Read the model definition and answer for the solid it produces. Units are mm, in the model's axes. Face numbers are marked on the shaded views. Coordinates: 2 decimals unless noted, no trailing zeros. Order: outer loops, then holes, each group sorted by start corner. A loop starts at its lowest first (then second) coordinate and runs counter-clockwise, first axis right, second up.
Autodesk Inventor part; units mm, degrees
ref_plane "YZ Plane" through (0, 0, 0) normal (1, 0, 0) x (0, 1, 0)
ref_plane "XZ Plane" through (0, 0, 0) normal (0, 1, 0) x (-1, 0, 0)
ref_plane "XY Plane" through (0, 0, 0) normal (0, 0, 1) x (1, 0, 0)
sketch "Sketch1" plane through (0, 0, 0) normal (0, 0, 1) x (1, 0, 0)
  line L0 (-3, 0) -> (3, 0) construction
  line L1 (-3, -1.5) -> (3, -1.5)
  line L2 (3, 1.5) -> (-3, 1.5)
  arc A0 (-3, 1.5) -> (-3, -1.5) centre (-3, 0) ccw
  arc A1 (3, -1.5) -> (3, 1.5) centre (3, 0) ccw
  point P0 (0, 0)
  point P1 (4.5, 0)
  point P2 (-4.5, 0)
  dimension "d0" = 3
  dimension "d1" = 9
extrude "Extrusion1" add sketch "Sketch1" along normal blind 7.5
sketch "Sketch2" plane through (-3, 1.5, 0) normal (0, 1, 0) x (1, 0, 0)
  line L0 (6, 0) -> (0, 0) construction
  line L1 (9, -15) -> (-3, -15)
  line L2 (-3, -15) -> (-3, -1)
  line L3 (-3, -1) -> (9, -1)
  line L4 (9, -1) -> (9, -15)
  line L5 (9, -15) -> (-3, -1) construction
  line L6 (-3, -15) -> (9, -1) construction
  point P0 (3, 0)
  point P1 (3, -8)
  point P2 (3, 0)
  dimension "d4" = 1
  dimension "d5" = 12
  dimension "d6" = 14
extrude "Extrusion2" add sketch "Sketch2" along normal blind 1
properties part number "usb" material "Acetal Resin, Black"
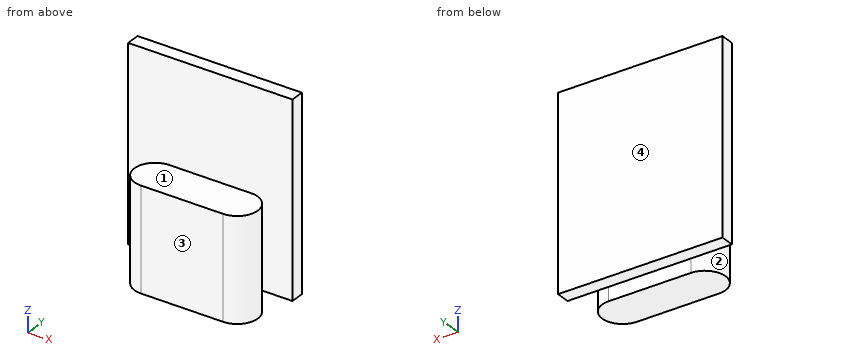
Q1. Straight lines are drawn through the part: L1, parallel to Z at x = 3.25, y = 0.75; L2, parallel to Y at x = 0, z = 9.5; L3, parallel to Z at x = 2.25, y = 2.15. For each, find the intervals that lie inside material, in ascending order.
Q2. The part is cut by section A-A, the plane x = -1.5. Determine the outline of the cut face in (y, z), then the cut area to 3 significant figures.
Q3. The part is cut by section B-B, the plane z = 6.25. Determine the outline of the cut face in (x, y), then the cut area to 3 significant figures.
Q4. Each of these flat-tipped pins is pushed along its axis until it touches: P1, Ø1.1, axis at x = 0, y = 2, coming from the -Z side; P2, Ø0.9, axis at x = -1, y = 0.5, coming from the +Z side. Where does it stop, or does it pass through?
Q5. The part is cut by section D-D, the plane z = 10.25. Determine the outline of the cut face in (x, y).
Q6. The part is cut by section C-C, the plane y = 0. Determine the outline of the cut face in (x, z), then the cut area to 3 significant figures.
Q7. Determine the mould class of the marked faces 1, 2, 3 and 4 for opening direction Y: +Y half, -Y half, draft (parallel to the pull), parting line (faces both ways), or undercut.
Computed values:
1. L1: z = 0 to 7.5
1. L2: y = 1.5 to 2.5
1. L3: z = 1 to 15
2. outline: (-1.5, 0) - (1.5, 0) - (1.5, 1) - (2.5, 1) - (2.5, 15) - (1.5, 15) - (1.5, 7.5) - (-1.5, 7.5) - close
2. area: 36.5 mm2
3. outline: (-6, 1.5) - (-3, 1.5) arc R1.5 ccw to (-3, -1.5) - (3, -1.5) arc R1.5 ccw to (3, 1.5) - (6, 1.5) - (6, 2.5) - (-6, 2.5) - close
3. area: 37.1 mm2
4. P1: stops at z = 0
4. P2: stops at z = 7.5
5. outline: (-6, 1.5) - (6, 1.5) - (6, 2.5) - (-6, 2.5) - close
6. outline: (-4.5, 0) - (4.5, 0) - (4.5, 7.5) - (-4.5, 7.5) - close
6. area: 67.5 mm2
7. face 1: draft
7. face 2: undercut
7. face 3: -Y half
7. face 4: +Y half
